Input: part model. Units: mm. Frame: model coordinates. Face numbers are marked on the shaded views. A direction names the side the tool comes from. Round coordinates to 2 decimals unless told otherwise and drop trailing zeros. Order: outer loops, then holes, each group sorted by start corner. A loop starts at its lowest first (then second) coordinate and runs counter-clockwise, first axis right, second up. Notation, with made-up numbers: (54.25, 56) -> (65.25, 56) arc R21 cw to (65.25, 93) -> close; hole circle Ø10 at (-5.5, -8.75). An arc over 180 degrees is marked (long way). Use a Markdown table: item, result.
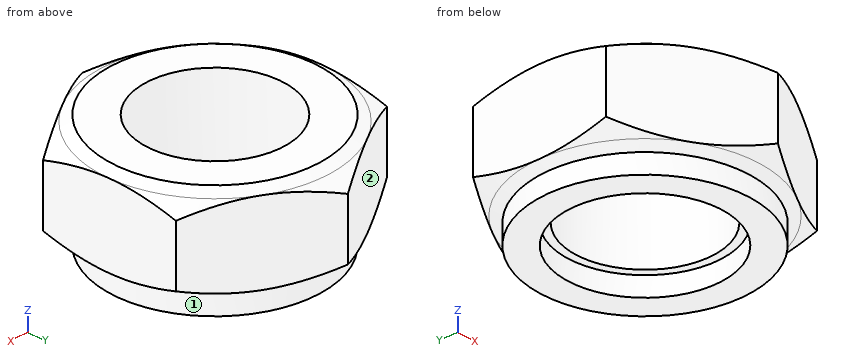
from build123d import *

# Parameters (mm, degrees)
EXTRUDE_1_DEPTH     = 4.8
SKETCH_3_R          = 7.25
CUT_EXTRUDE_1_DEPTH = 21.69202745
SKETCH_4_R          = 10.962716089
SKETCH_4_R_2        = 8.093789305
EXTRUDE_2_DEPTH     = 2


with BuildPart() as part:
    # 草图1 → 凸台-拉伸1 (new, symmetric)
    with BuildSketch(Plane.XY):
        Polygon((12, -6.92820323), (12, 6.92820323), (0, 13.856406461), (-12, 6.92820323), (-12, -6.92820323), (0, -13.856406461), align=None)
    extrude(amount=EXTRUDE_1_DEPTH, both=True)

    # 草图2 → 切除-旋转1 (revolve, cut)
    with BuildSketch(Plane(origin=(0, 0, 0), x_dir=(1, 0, 0), z_dir=(0, 1, 0))):
        Polygon((15.485203874, 8.108548082), (5.242876598, 8.108548082), (12, 4.2), (23.530399305, -2.469571859), align=None)
    cut_revolve_1 = revolve(axis=Axis((0, 0, -6.79329682), (0, 0, 1)), mode=Mode.SUBTRACT)

    # 镜向1: 切除-旋转1 across plane
    add(cut_revolve_1.mirror(Plane.XY), mode=Mode.SUBTRACT)

    # 草图3 → 切除-拉伸1 (cut, through all)
    with BuildSketch(Plane.XY.offset(4.8)):
        Circle(SKETCH_3_R)
    extrude(amount=-CUT_EXTRUDE_1_DEPTH, mode=Mode.SUBTRACT)

    # 草图4 → 凸台-拉伸2 (add)
    with BuildSketch(Plane(origin=(0, 0, -4.8), x_dir=(-1, 0, 0), z_dir=(0, 0, -1))):
        Circle(SKETCH_4_R)
        Circle(SKETCH_4_R_2, mode=Mode.SUBTRACT)
    extrude(amount=EXTRUDE_2_DEPTH)


solid = part.part
1) Ray query, probe 1 along Y at (x, z) = (0, -6); probe 2 along Z at (x, y) = (2, -7.5); probe 3 along X at (y, z) = (4, -4.25). Return the intervals inside material, ascending.
Answer key:
| item | result |
|---|---|
| probe 1 | y = -10.96 to -8.09, 8.09 to 10.96 |
| probe 2 | z = -4.8 to 4.8 |
| probe 3 | x = -11.22 to -6.05, 6.05 to 11.22 |
2) Contact query for a flat-ended pin moving along its axis: P1, Ø1, axis at x = -3, z = -2, coming from the -Y side. Output: stop coordinate, or through.
Answer key:
| item | result |
|---|---|
| P1 | stops at y = -12.41 |
3) Cut plane A-A on z = -2. Return loops of the section in (x, y), and give its area (3 significant figures).
Answer key:
| item | result |
|---|---|
| outline | (-12, -6.93) -> (0, -13.86) -> (12, -6.93) -> (12, 6.93) -> (0, 13.86) -> (-12, 6.93) -> close; hole circle Ø14.5 at (0, 0) |
| area | 334 mm^2 |
4) Set-up query: the marked faces 1 and 2. Return all of +Z, -Z, +X, -X, +Y, -Y with unobstructed straight access to the full face (end or side cutting, diameter ignored); none if empty.
Answer key:
| item | result |
|---|---|
| face 1 | -Z |
| face 2 | +Z, -Z, -X, +Y |
